Check sheet for the modelled part. Datum: model origin and axes. Units: mm. Coordinates: 2 decimals unless noted, no trailing zeros. Loops run counter-clockwise (first coordinate to the right, second up) from the corner with the lowest first, then second, coordinate; pieces in that order, holes last. Notation, with made-up numbers: M 65,56.25 L 93,56.25 A12 ccw 93,61.25 Z; hole C 46.25,70 d9. An arc over 180 degrees is marked long. Return JSON: item names as keys, results as strings.
Autodesk Inventor part; units mm, degrees
ref_plane "YZ Plane" through (0, 0, 0) normal (1, 0, 0) x (0, 1, 0)
ref_plane "XZ Plane" through (0, 0, 0) normal (0, 1, 0) x (-1, 0, 0)
ref_plane "XY Plane" through (0, 0, 0) normal (0, 0, 1) x (1, 0, 0)
sketch "Sketch1" plane through (0, 0, 0) normal (1, 0, 0) x (0, 1, 0)
  line L0 (46.7204, 78.4349) -> (-54.8796, 78.4349)
  line L1 (-54.8796, 78.4349) -> (-54.8796, -48.5651)
  line L2 (-54.8796, -48.5651) -> (46.7204, -48.5651)
  line L3 (46.7204, -48.5651) -> (46.7204, 78.4349)
  point P0 (0, 0)
  dimension "d0" = 127
  dimension "d1" = 101.6
extrude "Extrusion1" add sketch "Sketch1" along normal blind 6.35
sketch "Sketch2" plane through (6.35, 0, 0) normal (1, 0, 0) x (0, 0, -1)
  line L0 (48.5651, 46.7204) -> (-78.4349, 46.7204)
  line L1 (-78.4349, 46.7204) -> (-78.4349, -54.8796)
  line L2 (-78.4349, -54.8796) -> (48.5651, -54.8796)
  line L3 (48.5651, -54.8796) -> (48.5651, 46.7204)
  point P0 (0, 0)
  point P1 (-72.0849, 40.3704)
  point P2 (42.2151, 40.3704)
  point P3 (42.2151, -48.5296)
  point P4 (-72.0849, -48.5296)
  dimension "d4" = 0
  dimension "d5" = 0
  dimension "d6" = 0
  dimension "d7" = 0
  dimension "d8" = 6.35
  dimension "d9" = 6.35
  dimension "d10" = 6.35
  dimension "d11" = 6.35
hole "Hole1" at (6.35, 40.3704, 72.0849) at (6.35, 40.3704, -42.2151) at (6.35, -48.5296, -42.2151) at (6.35, -48.5296, 72.0849) direction (-1, 0, 0) diameter 4.318 end through all
sketch "Sketch3" plane through (6.35, 0, 0) normal (1, 0, 0) x (0, 0, -1)
  circle A0 centre (-46.6849, -23.1296) radius 9.652
  line L0 (-78.4349, -54.8796) -> (48.5651, -54.8796)
  line L1 (-78.4349, 46.7204) -> (-78.4349, -54.8796)
  point P0 (0, 0)
  dimension "d19" = 19.304
  dimension "d20" = 31.75
  dimension "d21" = 31.75
extrude "Extrusion2" cut sketch "Sketch3" against normal blind 61.9125
sketch "Sketch4" plane through (6.35, 0, 0) normal (1, 0, 0) x (0, 0, -1)
  circle A0 centre (-46.6849, -23.1296) radius 9.652
  circle A1 centre (-46.6849, -23.1296) radius 9.652
  circle A2 centre (-46.6849, -23.1296) radius 25.4
  line L0 (-46.6849, -23.1296) -> (-105.0514, -23.1296)
  line L1 (-46.6849, -23.1296) -> (-64.9089, 8.4353)
  line L2 (-46.6849, -23.1296) -> (-26.8908, 11.1548)
  line L3 (-46.6849, -23.1296) -> (1.7612, -23.1296)
  line L4 (-46.6849, -23.1296) -> (-29.0867, -53.6105)
  line L5 (-46.6849, -23.1296) -> (-67.8043, -59.7094)
  point P0 (0, 0)
  point P1 (-72.0849, -23.1296)
  point P2 (-21.2849, -23.1296)
  point P3 (-59.3849, -1.1326)
  point P4 (-33.9849, -1.1326)
  point P5 (-33.9849, -45.1267)
  point P6 (-59.3849, -45.1267)
  dimension "d24" = 50.8
  dimension "d25" = 60
  dimension "d26" = 60
  dimension "d27" = 60
  dimension "d28" = 60
hole "Hole2" at (6.35, -23.1296, 72.0849) at (6.35, -23.1296, 21.2849) at (6.35, -1.1326, 59.3849) at (6.35, -1.1326, 33.9849) at (6.35, -45.1267, 33.9849) at (6.35, -45.1267, 59.3849) direction (-1, 0, 0) diameter 4.318 end through all
sketch "Sketch5" plane through (6.35, 0, 0) normal (1, 0, 0) x (0, 0, -1)
  circle A0 centre (-14.6316, -0.2696) radius 11.1125
  circle A1 centre (-46.6849, -23.1296) radius 9.652
  circle A2 centre (-46.6849, -23.1296) radius 39.37
  point P0 (0, 0)
  dimension "d37" = 78.74
  dimension "d36" = 22.225
  dimension "d44" = 22.86
extrude "Extrusion3" cut sketch "Sketch5" against normal blind 66.675 contours A0 A2 | A2 A0 picked at (-11.8926, 2.0476) picked at (-17.7425, -2.4882)
sketch "Sketch6" plane through (6.35, 0, 0) normal (1, 0, 0) x (0, 0, -1)
  circle A0 centre (-14.6316, -0.2696) radius 11.1125
  circle A1 centre (-14.6316, -0.2696) radius 40.64
  circle A2 centre (10.7367, -32.0196) radius 14.2748
  line L0 (48.5651, 46.7204) -> (-78.4349, 46.7204)
  point P0 (0, 0)
  dimension "d43" = 81.28
  dimension "d40" = 28.5496
  dimension "d76" = 78.74
extrude "Extrusion4" cut sketch "Sketch6" against normal blind 39.6875 contours A2 A1 | A1 A2 picked at (11.4749, -25.7156) picked at (9.3568, -38.0591)
properties part number "OutsideMotorPlate" material "Aluminum 6061"
1) Section check C-C on x = 1. Count the separate pieces of the cut face and the enclosed holes in it, then the cut area to 3 significant figures.
Answers:
{"separate pieces": "1", "enclosed holes": "13", "area": "11,400 mm²"}
2) Draft check along Y on faces 1 (the face through (3.131, -49.989, 73.676)), 2 (the face through (3.131, -23.225, 74.242)), 3 (the face through (3, -5, -48.565)), 4 (the face through (3, 46.72, 14)). Enter one of: +Y half, -Y half, draft (parallel to the pull), parting line (faces both ways), or undercut.
Answers:
{"face 1": "undercut", "face 2": "undercut", "face 3": "draft", "face 4": "+Y half"}
3) Scan lines: line 1 along Z through (x, y) = (5.75, -21.5); line 2 along Z through (x, y) = (6.25, -48.5); line 3 along Z through (x, y) = (4.75, -29.5). Record each from-to range of solid material in increasing order. Write a range as [from, to].
Answers:
{"line 1": "[-48.57, -20.39], [-1.09, 19.87], [22.7, 37.17], [56.2, 70.67], [73.5, 78.43]", "line 2": "[-48.57, -44.37], [-40.06, 69.93], [74.24, 78.43]", "line 3": "[-48.57, -24.79], [3.31, 39.43], [53.94, 78.43]"}
4) Section check B-B on z = -9. Record the cut outline in (x, y).
Answers:
{"outline": "M 0,-54.88 L 6.35,-54.88 L 6.35,-46.19 L 0,-46.19 Z; M 0,-17.85 L 6.35,-17.85 L 6.35,46.72 L 0,46.72 Z"}
5) Go/stop test with a flat-tipped pin: pin 1 Ø2.5 at (y, z) = (-48.53, -42.22) entering from +X (1 decimal). Record where the tip stops, or that it passes through.
Answers:
{"pin 1": "through"}
6) Section check A-A on y = -6. Record the cut outline in (x, z).
Answers:
{"outline": "M 0,-48.57 L 6.35,-48.57 L 6.35,5.11 L 0,5.11 Z; M 0,24.15 L 6.35,24.15 L 6.35,78.43 L 0,78.43 Z"}
